```python
from build123d import *

# Parameters (mm, degrees)
EXTRUDE4_DEPTH = 12.7


with BuildPart() as part:
    # Sketch9 → Extrude4 (new body)
    with BuildSketch(Plane(origin=(0, 0, 0), x_dir=(1, 0, 0), z_dir=(0, 1, 0))):
        with BuildLine():
            Line((20.495684684, 31.492994432), (27.472430394, 43.577072472))
            ThreePointArc((27.472430394, 43.577072472), (30.531314315, 45.773497268), (34.201168909, 44.928973738))
            ThreePointArc((34.201168909, 44.928973738), (56.465322419, 0), (34.201168909, -44.928973738))
            ThreePointArc((34.201168909, -44.928973738), (30.531314315, -45.773497268), (27.472430394, -43.577072472))
            Line((27.472430394, -43.577072472), (20.495684684, -31.492994432))
            ThreePointArc((20.495684684, -31.492994432), (19.333554027, -30.330863775), (17.746054027, -29.905494432))
            Line((17.746054027, -29.905494432), (-21.795601412, -29.905494432))
            ThreePointArc((-21.795601412, -29.905494432), (-26.285729472, -28.045622492), (-28.145601412, -23.555494432))
            Line((-28.145601412, -23.555494432), (-28.145601412, 23.555494432))
            ThreePointArc((-28.145601412, 23.555494432), (-26.285729472, 28.045622492), (-21.795601412, 29.905494432))
            Line((-21.795601412, 29.905494432), (17.746054027, 29.905494432))
            ThreePointArc((17.746054027, 29.905494432), (19.333554027, 30.330863775), (20.495684684, 31.492994432))
        make_face()
    extrude(amount=-EXTRUDE4_DEPTH)


solid = part.part
```
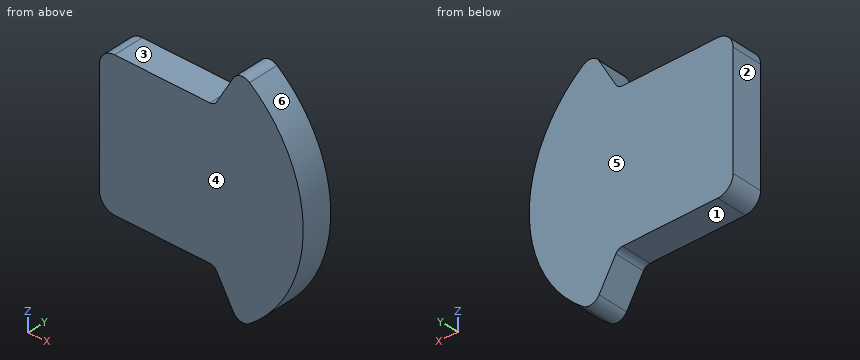
Input: part model. Units: mm. Frame: model coordinates. Face numbers are marked on the shaded views. A direction names the side the tool comes from. Round coordinates to 2 decimals unless told otherwise and drop trailing zeros. Write each loop counter-clockwise with the first axis right and the second up, starting at its lowest first coordinate (ties: lowest second). Pieces come first, ordered by that corner, then holes. Notation, with made-up numbers: (48, 88.25) -> (76, 88.25) arc R18 cw to (76, 117.25) -> close; hole circle Ø5 at (-7, 87.25). An arc over 180 degrees is marked (long way). Answer as CSV lines item,"result".
1. Ray query, L1, parallel to Z at x = -13, y = -1.25; L2, parallel to Z at x = 37, y = -7.75; L3, parallel to X at y = -11.25, z = -23. Return the intervals inside material, ascending. Write a range as [from, to].
Geometry says:
L1,"z = [-29.91, 29.91]"
L2,"z = [-42.65, 42.65]"
L3,"x = [-28.15, 51.57]"
2. Reachability of the marked faces 1, 2 and 3 from +Z, -Z, +X, -X, +Y, -Y: full face, straight path, thin tool, end or side. Return the list, or none.
Geometry says:
face 1,"-Z, -X, +Y, -Y"
face 2,"+Z, -Z, -X, +Y, -Y"
face 3,"+Z, -X, +Y, -Y"
3. Contact query for flat-ended pins moving along their axis: P1, Ø2, axis at y = -7, z = -24.5, coming from the +X side; P2, Ø6.5, axis at x = -7.5, y = -4, coming from the -Z side; P3, Ø5, axis at x = -7, y = -3, coming from the +Z side; P4, Ø12, axis at x = 21.5, z = 2.5, coming from the +Y side. Output: stop coordinate, or through.
Geometry says:
P1,"stops at x = 51.34"
P2,"stops at z = -29.91"
P3,"stops at z = 29.91"
P4,"stops at y = 0"
4. Section B-B (x = 5.5). Return the cut outline in (y, z), plus the area to 3 significant figures.
Geometry says:
outline,"(-12.7, -29.91) -> (0, -29.91) -> (0, 29.91) -> (-12.7, 29.91) -> close"
area,"760 mm^2"
5. Section C-C (z = 33.5). Return the cut outline in (x, y), plus the area to 3 significant figures.
Geometry says:
outline,"(21.65, -12.7) -> (45.45, -12.7) -> (45.45, 0) -> (21.65, 0) -> close"
area,"302 mm^2"
6. Mould query, pull axis Y, two halves, no side actions, for the marked faces 4, 5 and 6. Classes: +Y half, -Y half, draft (parallel to the pull), parting line (faces both ways), or undercut.
Geometry says:
face 4,"-Y half"
face 5,"+Y half"
face 6,"draft"
